from build123d import *

# Parameters (mm, degrees)
F1_DEPTH = 2
F2_R     = 1
F3_DEPTH = 2.001


with BuildPart() as f1:
    # F0 (on Top) → F1 (new body)
    with BuildSketch(Plane.XY):
        with BuildLine():
            ThreePointArc((7.420617, -1.088319), (7.480128, -0.545605), (7.5, 0))
            ThreePointArc((7.5, 0), (7.480128, 0.545605), (7.420617, 1.088319))
            ThreePointArc((7.420617, 1.088319), (7.35589, 1.463177), (7.272238, 1.834271))
            ThreePointArc((7.272238, 1.834271), (6.929096, 2.870126), (6.439275, 3.845223))
            ThreePointArc((6.439275, 3.845223), (6.236022, 4.166777), (6.016727, 4.477611))
            ThreePointArc((6.016727, 4.477611), (5.303301, 5.303301), (4.477611, 6.016727))
            ThreePointArc((4.477611, 6.016727), (4.166777, 6.236022), (3.845223, 6.439275))
            ThreePointArc((3.845223, 6.439275), (2.870126, 6.929096), (1.834271, 7.272238))
            ThreePointArc((1.834271, 7.272238), (1.463177, 7.35589), (1.088319, 7.420617))
            ThreePointArc((1.088319, 7.420617), (0, 7.5), (-1.088319, 7.420617))
            ThreePointArc((-1.088319, 7.420617), (-1.463177, 7.35589), (-1.834271, 7.272238))
            ThreePointArc((-1.834271, 7.272238), (-2.870126, 6.929096), (-3.845223, 6.439275))
            ThreePointArc((-3.845223, 6.439275), (-4.166777, 6.236022), (-4.477611, 6.016727))
            ThreePointArc((-4.477611, 6.016727), (-5.303301, 5.303301), (-6.016727, 4.477611))
            ThreePointArc((-6.016727, 4.477611), (-6.236022, 4.166777), (-6.439275, 3.845223))
            ThreePointArc((-6.439275, 3.845223), (-6.929096, 2.870126), (-7.272238, 1.834271))
            ThreePointArc((-7.272238, 1.834271), (-7.35589, 1.463177), (-7.420617, 1.088319))
            ThreePointArc((-7.420617, 1.088319), (-7.5, 0), (-7.420617, -1.088319))
            ThreePointArc((-7.420617, -1.088319), (-7.35589, -1.463177), (-7.272238, -1.834271))
            ThreePointArc((-7.272238, -1.834271), (-6.929096, -2.870126), (-6.439275, -3.845223))
            ThreePointArc((-6.439275, -3.845223), (-6.236022, -4.166777), (-6.016727, -4.477611))
            ThreePointArc((-6.016727, -4.477611), (-5.303301, -5.303301), (-4.477611, -6.016727))
            ThreePointArc((-4.477611, -6.016727), (-4.166777, -6.236022), (-3.845223, -6.439275))
            ThreePointArc((-3.845223, -6.439275), (-2.870126, -6.929096), (-1.834271, -7.272238))
            ThreePointArc((-1.834271, -7.272238), (-1.463177, -7.35589), (-1.088319, -7.420617))
            ThreePointArc((-1.088319, -7.420617), (0, -7.5), (1.088319, -7.420617))
            ThreePointArc((1.088319, -7.420617), (1.463177, -7.35589), (1.834271, -7.272238))
            ThreePointArc((1.834271, -7.272238), (2.870126, -6.929096), (3.845223, -6.439275))
            ThreePointArc((3.845223, -6.439275), (4.166777, -6.236022), (4.477611, -6.016727))
            ThreePointArc((4.477611, -6.016727), (5.303301, -5.303301), (6.016727, -4.477611))
            ThreePointArc((6.016727, -4.477611), (6.236022, -4.166777), (6.439275, -3.845223))
            ThreePointArc((6.439275, -3.845223), (6.929096, -2.870126), (7.272238, -1.834271))
            ThreePointArc((7.272238, -1.834271), (7.35589, -1.463177), (7.420617, -1.088319))
        make_face()
        with BuildLine():
            ThreePointArc((7.420617, 1.088319), (7.480128, 0.545605), (7.5, 0))
            ThreePointArc((7.5, 0), (7.480128, -0.545605), (7.420617, -1.088319))
            ThreePointArc((7.420617, -1.088319), (8.504352, -0.949828), (9.5, -0.5))
            Line((9.5, -0.5), (9.5, 0))
            Line((9.5, 0), (9.5, 0.5))
            ThreePointArc((9.5, 0.5), (8.504352, 0.949828), (7.420617, 1.088319))
        make_face()
        with BuildLine():
            ThreePointArc((6.439275, 3.845223), (6.929096, 2.870126), (7.272238, 1.834271))
            ThreePointArc((7.272238, 1.834271), (8.22048, 2.376948), (8.968197, 3.173553))
            Line((8.968197, 3.173553), (8.776856, 3.635493))
            Line((8.776856, 3.635493), (8.585514, 4.097432))
            ThreePointArc((8.585514, 4.097432), (7.493513, 4.132001), (6.439275, 3.845223))
        make_face()
        with BuildLine():
            ThreePointArc((8.968197, -3.173553), (8.22048, -2.376948), (7.272238, -1.834271))
            ThreePointArc((7.272238, -1.834271), (6.929096, -2.870126), (6.439275, -3.845223))
            ThreePointArc((6.439275, -3.845223), (7.493513, -4.132001), (8.585514, -4.097432))
            Line((8.585514, -4.097432), (8.776856, -3.635493))
            Line((8.776856, -3.635493), (8.968197, -3.173553))
        make_face()
        with BuildLine():
            ThreePointArc((4.477611, 6.016727), (5.303301, 5.303301), (6.016727, 4.477611))
            ThreePointArc((6.016727, 4.477611), (6.685115, 5.341855), (7.071068, 6.363961))
            Line((7.071068, 6.363961), (6.717514, 6.717514))
            Line((6.717514, 6.717514), (6.363961, 7.071068))
            ThreePointArc((6.363961, 7.071068), (5.341855, 6.685115), (4.477611, 6.016727))
        make_face()
        with BuildLine():
            ThreePointArc((7.071068, -6.363961), (6.685115, -5.341855), (6.016727, -4.477611))
            ThreePointArc((6.016727, -4.477611), (5.303301, -5.303301), (4.477611, -6.016727))
            ThreePointArc((4.477611, -6.016727), (5.341855, -6.685115), (6.363961, -7.071068))
            Line((6.363961, -7.071068), (6.717514, -6.717514))
            Line((6.717514, -6.717514), (7.071068, -6.363961))
        make_face()
        with BuildLine():
            ThreePointArc((1.834271, 7.272238), (2.870126, 6.929096), (3.845223, 6.439275))
            ThreePointArc((3.845223, 6.439275), (4.132001, 7.493513), (4.097432, 8.585514))
            Line((4.097432, 8.585514), (3.635493, 8.776856))
            Line((3.635493, 8.776856), (3.173553, 8.968197))
            ThreePointArc((3.173553, 8.968197), (2.376948, 8.22048), (1.834271, 7.272238))
        make_face()
        with BuildLine():
            ThreePointArc((4.097432, -8.585514), (4.132001, -7.493513), (3.845223, -6.439275))
            ThreePointArc((3.845223, -6.439275), (2.870126, -6.929096), (1.834271, -7.272238))
            ThreePointArc((1.834271, -7.272238), (2.376948, -8.22048), (3.173553, -8.968197))
            Line((3.173553, -8.968197), (3.635493, -8.776856))
            Line((3.635493, -8.776856), (4.097432, -8.585514))
        make_face()
        with BuildLine():
            ThreePointArc((-1.088319, 7.420617), (0, 7.5), (1.088319, 7.420617))
            ThreePointArc((1.088319, 7.420617), (0.949828, 8.504352), (0.5, 9.5))
            Line((0.5, 9.5), (0, 9.5))
            Line((0, 9.5), (-0.5, 9.5))
            ThreePointArc((-0.5, 9.5), (-0.949828, 8.504352), (-1.088319, 7.420617))
        make_face()
        with BuildLine():
            ThreePointArc((0.5, -9.5), (0.949828, -8.504352), (1.088319, -7.420617))
            ThreePointArc((1.088319, -7.420617), (0, -7.5), (-1.088319, -7.420617))
            ThreePointArc((-1.088319, -7.420617), (-0.949828, -8.504352), (-0.5, -9.5))
            Line((-0.5, -9.5), (0, -9.5))
            Line((0, -9.5), (0.5, -9.5))
        make_face()
        with BuildLine():
            ThreePointArc((-3.845223, 6.439275), (-2.870126, 6.929096), (-1.834271, 7.272238))
            ThreePointArc((-1.834271, 7.272238), (-2.376948, 8.22048), (-3.173553, 8.968197))
            Line((-3.173553, 8.968197), (-3.635493, 8.776856))
            Line((-3.635493, 8.776856), (-4.097432, 8.585514))
            ThreePointArc((-4.097432, 8.585514), (-4.132001, 7.493513), (-3.845223, 6.439275))
        make_face()
        with BuildLine():
            ThreePointArc((-3.173553, -8.968197), (-2.376948, -8.22048), (-1.834271, -7.272238))
            ThreePointArc((-1.834271, -7.272238), (-2.870126, -6.929096), (-3.845223, -6.439275))
            ThreePointArc((-3.845223, -6.439275), (-4.132001, -7.493513), (-4.097432, -8.585514))
            Line((-4.097432, -8.585514), (-3.635493, -8.776856))
            Line((-3.635493, -8.776856), (-3.173553, -8.968197))
        make_face()
        with BuildLine():
            ThreePointArc((-6.016727, 4.477611), (-5.303301, 5.303301), (-4.477611, 6.016727))
            ThreePointArc((-4.477611, 6.016727), (-5.341855, 6.685115), (-6.363961, 7.071068))
            Line((-6.363961, 7.071068), (-6.717514, 6.717514))
            Line((-6.717514, 6.717514), (-7.071068, 6.363961))
            ThreePointArc((-7.071068, 6.363961), (-6.685115, 5.341855), (-6.016727, 4.477611))
        make_face()
        with BuildLine():
            ThreePointArc((-6.363961, -7.071068), (-5.341855, -6.685115), (-4.477611, -6.016727))
            ThreePointArc((-4.477611, -6.016727), (-5.303301, -5.303301), (-6.016727, -4.477611))
            ThreePointArc((-6.016727, -4.477611), (-6.685115, -5.341855), (-7.071068, -6.363961))
            Line((-7.071068, -6.363961), (-6.717514, -6.717514))
            Line((-6.717514, -6.717514), (-6.363961, -7.071068))
        make_face()
        with BuildLine():
            ThreePointArc((-7.272238, 1.834271), (-6.929096, 2.870126), (-6.439275, 3.845223))
            ThreePointArc((-6.439275, 3.845223), (-7.493513, 4.132001), (-8.585514, 4.097432))
            Line((-8.585514, 4.097432), (-8.776856, 3.635493))
            Line((-8.776856, 3.635493), (-8.968197, 3.173553))
            ThreePointArc((-8.968197, 3.173553), (-8.22048, 2.376948), (-7.272238, 1.834271))
        make_face()
        with BuildLine():
            ThreePointArc((-8.585514, -4.097432), (-7.493513, -4.132001), (-6.439275, -3.845223))
            ThreePointArc((-6.439275, -3.845223), (-6.929096, -2.870126), (-7.272238, -1.834271))
            ThreePointArc((-7.272238, -1.834271), (-8.22048, -2.376948), (-8.968197, -3.173553))
            Line((-8.968197, -3.173553), (-8.776856, -3.635493))
            Line((-8.776856, -3.635493), (-8.585514, -4.097432))
        make_face()
        with BuildLine():
            ThreePointArc((-7.420617, -1.088319), (-7.5, 0), (-7.420617, 1.088319))
            ThreePointArc((-7.420617, 1.088319), (-8.504352, 0.949828), (-9.5, 0.5))
            Line((-9.5, 0.5), (-9.5, 0))
            Line((-9.5, 0), (-9.5, -0.5))
            ThreePointArc((-9.5, -0.5), (-8.504352, -0.949828), (-7.420617, -1.088319))
        make_face()
    extrude(amount=F1_DEPTH)

    # F2 (on face) → F3 (cut, through all)
    with BuildSketch(Plane.XY.offset(2)):
        Circle(F2_R)
    extrude(amount=-F3_DEPTH, mode=Mode.SUBTRACT)


solid = f1.part
Read the model definition and answer for the solid it produces. Units are mm, in the model's axes. A direction names the side the tool comes from. Give positions to 0.01 mm unless a question says otherwise; leave off trailing zeros. Loops run counter-clockwise (first coordinate to the right, second up) from the corner with the lowest first, then second, coordinate; pieces in that order, holes last. Notation, with made-up numbers: (13.5, 44.5) - (53.5, 44.5) arc R21 cw to (53.5, 59.5) - close; hole circle Ø11 at (-8.5, 32). An arc over 180 degrees is marked (long way). Answer as CSV lines item,"result". Start each with the question number.
1) Find section A-A (y = 0). Write down the section's boundary in (x, z), then the cut area to 3 significant figures.
2) Determine the mould class of faces 1 (the face through (0, -2, 2)), 2 (the face through (5.33, -6.68, 0.99)), 3 (the face through (8.21, 2.37, 0.99)) for opening direction Y: released by +Y, released by -Y, zero draft, split by the parting line, or undercut.
3) Find section C-C (x = 5.75). Write down the section's boundary in (y, z), then the cut area to 3 significant figures.
4) This flat-tipped pin is pushed along its axis until it touches: pin 1 Ø1.8 at (x, y) = (0, 0) entering from -Z. Where does it stop, or does it pass through?
5) Which of the six approach directions +Z, -Z, +X, -X, +Y, -Y give full straight-line access (tool end or side, diameter ignored) to faces 4 (the face through (6.68, 5.33, 0.99)), 5 (the face through (-5.33, 6.68, 0.99)), 6 (the face through (4.134, -7.509, 0.986)), 7 (the face through (0, -2, 0)), 8 (the face through (-8.233, 2.386, 0.986))?
6) Straight lines are drawn through the part: L1, parallel to Y at x = 0, z = 1.1; L2, parallel to Y at x = 6.75, z = 0.6; L3, parallel to X at y = 8, z = 1.1. For each, find the intervals that lie inside material, in ascending order. Write a range as from..to.
Findings below:
1,outline,"(-9.5, 0) - (-1, 0) - (-1, 2) - (-9.5, 2) - close; (1, 0) - (9.5, 0) - (9.5, 2) - (1, 2) - close"
1,area,"34.0 mm^2"
2,face 1,"zero draft"
2,face 2,"released by -Y"
2,face 3,"undercut"
3,outline,"(-6.88, 0) - (6.88, 0) - (6.88, 2) - (-6.88, 2) - close"
3,area,"27.5 mm^2"
4,pin 1,"through"
5,face 4,"+Z, -Z, +X"
5,face 5,"+Z, -Z, +Y"
5,face 6,"+Z, -Z"
5,face 7,"-Z, +X, -X, +Y, -Y"
5,face 8,"+Z, -Z, -X"
6,L1,"-9.5..-1, 1..9.5"
6,L2,"-6.69..-5.46, -3.97..3.97, 5.46..6.69"
6,L3,"-4.16..-2.22, -1.06..1.06, 2.22..4.16"
